```python
from build123d import *

# Parameters (mm, degrees)
SKETCH1_W           = 25.4
SKETCH1_H           = 76.2
SKETCH1_R           = 2.5
BOSS_EXTRUDE1_DEPTH = 5
BOSS_EXTRUDE2_START = 38.1
SKETCH3_W           = 25.4
SKETCH3_H           = 25
SKETCH3_R           = 2.5
BOSS_EXTRUDE2_DEPTH = 5
BOSS_EXTRUDE3_START = -33.1
SKETCH3_5_W         = 25.4
SKETCH3_5_H         = 25
SKETCH3_5_R         = 2.5
BOSS_EXTRUDE3_DEPTH = 5
CUT_EXTRUDE1_START  = -3
CUT_EXTRUDE1_DEPTH  = 72.2
SKETCH5_R           = 2.5
BOSS_EXTRUDE4_DEPTH = 30
CUT_EXTRUDE2_DEPTH  = 3
SKETCH7_W           = 4
SKETCH7_H           = 10
SKETCH7_W_2         = 30
SKETCH7_H_2         = 4
SKETCH7_W_3         = 3
SKETCH7_H_3         = 9.256727868
BOSS_EXTRUDE5_DEPTH = 2.5
CHAMFER1_SIZE       = 2


with BuildPart() as part:
    # Sketch1 → Boss-Extrude1 (new body)
    with BuildSketch(Plane.XY):
        Rectangle(SKETCH1_W, SKETCH1_H)
        with Locations((0, 11.68)):
            Circle(SKETCH1_R, mode=Mode.SUBTRACT)
    extrude(amount=BOSS_EXTRUDE1_DEPTH)

    # Sketch3 → Boss-Extrude2 (add)
    with BuildSketch(Plane(origin=(0, 0, 0), x_dir=(1, 0, 0), z_dir=(0, 1, 0)).offset(BOSS_EXTRUDE2_START)):
        with Locations((0, -17.5)):
            Rectangle(SKETCH3_W, SKETCH3_H)
        with Locations(Location((0, -19.304, 0), (0, 0, 90))):
            Circle(SKETCH3_R, mode=Mode.SUBTRACT)
    extrude(amount=-BOSS_EXTRUDE2_DEPTH)

    # Sketch3<5> → Boss-Extrude3 (add)
    with BuildSketch(Plane(origin=(0, 0, 0), x_dir=(1, 0, 0), z_dir=(0, 1, 0)).offset(BOSS_EXTRUDE3_START)):
        with Locations((0, -17.5)):
            Rectangle(SKETCH3_5_W, SKETCH3_5_H)
        with Locations(Location((0, -19.304, 0), (0, 0, 90))):
            Circle(SKETCH3_5_R, mode=Mode.SUBTRACT)
    extrude(amount=-BOSS_EXTRUDE3_DEPTH)

    # Sketch4 → Cut-Extrude1 (cut)
    with BuildSketch(Plane.XZ.offset(-33.1).offset(CUT_EXTRUDE1_START)):
        Polygon((2.367136104, 15.204), (4.734272207, 19.304), (2.367136104, 23.404), (-2.367136104, 23.404), (-4.734272207, 19.304), (-2.367136104, 15.204), align=None)
    extrude(amount=CUT_EXTRUDE1_DEPTH, mode=Mode.SUBTRACT)

    # Sketch5 → Boss-Extrude4 (add)
    with BuildSketch(Plane.XY.offset(5)):
        with Locations((0, -16.479)):
            Circle(SKETCH5_R)
        Polygon((-2.9, -12.279), (2.9, -12.279), (5.85, -9.329), (5.85, -8.379), (2.9, -8.379), (2.9, -6.479), (-2.9, -6.479), (-2.9, -8.379), (-5.85, -8.379), (-5.85, -9.329), align=None)
        Polygon((4.2, -13.579), (4.2, -19.379), (7.15, -22.329), (8.1, -22.329), (8.1, -19.379), (10, -19.379), (10, -13.579), (8.1, -13.579), (8.1, -10.629), (7.15, -10.629), align=None)
        Polygon((2.9, -20.679), (-2.9, -20.679), (-5.85, -23.629), (-5.85, -24.579), (-2.9, -24.579), (-2.9, -26.479), (2.9, -26.479), (2.9, -24.579), (5.85, -24.579), (5.85, -23.629), align=None)
        Polygon((-4.2, -19.379), (-4.2, -13.579), (-7.15, -10.629), (-8.1, -10.629), (-8.1, -13.579), (-10, -13.579), (-10, -19.379), (-8.1, -19.379), (-8.1, -22.329), (-7.15, -22.329), align=None)
    extrude(amount=BOSS_EXTRUDE4_DEPTH)

    # Sketch6 → Cut-Extrude2 (cut)
    with BuildSketch(Plane.XY.offset(5)):
        Polygon((2.367136104, 7.58), (4.734272207, 11.68), (2.367136104, 15.78), (-2.367136104, 15.78), (-4.734272207, 11.68), (-2.367136104, 7.58), align=None)
    extrude(amount=-CUT_EXTRUDE2_DEPTH, mode=Mode.SUBTRACT)

    # Sketch7 → Boss-Extrude5 (add, symmetric)
    with BuildSketch(Plane(origin=(0, 0, 0), x_dir=(0, 0, -1), z_dir=(1, 0, 0))):
        with Locations((-32, 33.1)):
            Rectangle(SKETCH7_W, SKETCH7_H)
        with Locations((-49, 30.1)):
            Rectangle(SKETCH7_W_2, SKETCH7_H_2)
        with Locations((-65.5, 32.728363934)):
            Rectangle(SKETCH7_W_3, SKETCH7_H_3)
    extrude(amount=BOSS_EXTRUDE5_DEPTH, both=True)

    # Chamfer1
    chamfer1_edges = [part.edges().sort_by_distance(p)[0] for p in [
        (0, 33.1, 30),
        (0, 32.1, 34),
    ]]
    chamfer(chamfer1_edges, length=CHAMFER1_SIZE)


solid = part.part
```
The model under review builds one solid part; all positions refer to its coordinate system, in mm. A direction names the side the tool comes from. Round coordinates to 2 decimals unless told otherwise and drop trailing zeros. Loops run counter-clockwise (first coordinate to the right, second up) from the corner with the lowest first, then second, coordinate; pieces in that order, holes last.
Item 1: Take a section at A-A (x = -11). Write out the cut boundary in (y, z).
Determined:
outline: (-38.1, 0) - (38.1, 0) - (38.1, 30) - (33.1, 30) - (33.1, 5) - (-33.1, 5) - (-33.1, 30) - (-38.1, 30) - close
Item 2: For faces 5 (the face through (8, 36, 30)), 6 (the face through (-2.9, -26, 20)), 7 (the face through (8.1, -12, 20)), 8 (the face through (-3.534, 34.621, 21.383)), 9 (the face through (0, -12.279, 20)), list the 3-axis set-ups (+Z, -Z, +X, -X, +Y, -Y) from which the entire face can be reached by the end or side of a thin tool; tool diameter is ignored.
Determined:
face 5: +Z, +X, +Y
face 6: +Z, -X
face 7: +Z, +X
face 8: none
face 9: +Z
Item 3: Take a section at C-C (x = 0). Give the number of separate pieces and of enclosed holes in the cut face, then the cut area to 3 significant figures.
Determined:
separate pieces: 4
enclosed holes: 0
area: 1,220 mm2
Item 4: Take a section at B-B (y = 24). Write out the cut boundary in (x, z).
Determined:
outline: (-12.7, 0) - (12.7, 0) - (12.7, 5) - (-12.7, 5) - close
Item 5: Clearance check with flat-ended pins moving along their axes: pin 1 Ø8 at (x, z) = (4, 53.5) entering from +Y; pin 2 Ø4 at (x, z) = (-0.5, 49) entering from -Y; pin 3 Ø0.8 at (y, z) = (-9, 24.5) entering from -X. State where each tip first meets the part, or that it passes through.
Determined:
pin 1: stops at y = 32.1
pin 2: stops at y = 28.1
pin 3: stops at x = -5.85
Item 6: Take a section at D-D (z = 61). Write out the cut boundary in (x, y), then the cut area to 3 significant figures.
Determined:
outline: (-2.5, 28.1) - (2.5, 28.1) - (2.5, 32.1) - (-2.5, 32.1) - close
area: 20.0 mm2
Item 7: For line 1 (Y direction, x = 8.75, z = 21); line 2 (Z direction, x = -1.5, y = 34); line 3 (Y direction, x = 6, z = 19), list the stretches that pass through material, from the lowest coordinate up.
Determined:
line 1: y = -38.1 to -33.1, -19.38 to -13.58, 33.1 to 38.1
line 2: z = 0 to 15.2, 23.4 to 34.1, 64 to 67
line 3: y = -38.1 to -33.1, -21.18 to -11.78, 33.1 to 38.1
Item 8: Mouldability with a two-part tool opening along Z and no side actions: class faces 1 (the face through (0, 35, 15.204)), 2 (the face through (0, 35, 64)), 3 (the face through (0, -16, 35)), 4 (the face through (-4, -24.579, 20)) as released by +Z, released by -Z, zero draft, split by the parting line, or undercut.
Determined:
face 1: undercut
face 2: undercut
face 3: released by +Z
face 4: zero draft
